Check sheet for the modelled part. Datum: model origin and axes. Units: mm. A direction names the side the tool comes from. Round coordinates to 2 decimals unless told otherwise and drop trailing zeros. Order: outer loops, then holes, each group sorted by start corner. A loop starts at its lowest first (then second) coordinate and runs counter-clockwise, first axis right, second up. Notation, with made-up numbers: M 55.5,-39.5 L 75.5,-39.5 A28 ccw 75.5,-19.5 Z; hole C 69,54 d7. An arc over 180 degrees is marked long. One line per item, written item: value. Start each with the question number.
(1) Access from +Z, -Z, +X, -X, +Y, -Y to the whole of each face (thin tool, end or side, straight path). Record for faces 1 (the face through (18, 24, 25)), 2 (the face through (9, 23, 12)).
(2) Depth check by flat-ended pin: pin 1 Ø3 at (x, y) = (19.5, 22.5) entering from +Z; pin 2 Ø7 at (x, z) = (6.5, 12) entering from -Y; pin 3 Ø8 at (y, z) = (12, 14) entering from -X; pin 4 Ø5 at (x, y) = (9, 19.5) entering from -Z. Enter the tip coordinate at first touch or a pass-through.
(3) Cross-section at B-B, the plane x = 12.5. Enter the section's corners in (y, z), and give its area (3 significant figures).
(4) Cross-section at A-A, the plane z = 12.5. Enter the section's corners in (x, y), and give its area (3 significant figures).
(5) Cross-section at D-D, the plane z = 2. Enter the section's corners in (x, y).
(6) Thickness scan on L1, parallel to Z at x = 12.5, y = 23.6; L2, parallel to Y at x = 13, z = 14.5. Record the ranges inside material, lowest first.
(7) Release check for a two-part mould opening along Z. For faces 3 (the face through (12.76, 24.014, 14.483)), 4 (the face through (23, 9, 12)), 5 (the face through (18, 24, 0)) record: released by +Z, released by -Z, zero draft, split by the parting line, or undercut.
from build123d import *

# Parameters (mm, degrees)
F1_DEPTH = 25
F2_R     = 2
F3_DEPTH = 25.001
F4_R     = 2
F5_DEPTH = 25.001


with BuildPart() as f1:
    # F0 (on Top) → F1 (new body)
    with BuildSketch(Plane.XY):
        Polygon((23, 23), (23, 0), (25, 0), (25, 25), (0, 25), (0, 23), align=None)
    extrude(amount=F1_DEPTH)

    # F2 (on face) → F3 (cut, through all)
    with BuildSketch(Plane(origin=(0, 25, 0), x_dir=(-1, 0, 0), z_dir=(0, 1, 0))):
        with Locations((-12.5, 12.5)):
            Circle(F2_R)
    extrude(amount=-F3_DEPTH, mode=Mode.SUBTRACT)

    # F4 (on face) → F5 (cut, through all)
    with BuildSketch(Plane.YZ.offset(25)):
        with Locations((12.5, 12.5)):
            Circle(F4_R)
    extrude(amount=-F5_DEPTH, mode=Mode.SUBTRACT)


solid = f1.part
Values found:
1. face 1: +Z, +X, -X, +Y, -Y
1. face 2: +Z, -Z, -X, -Y
2. pin 1: z = 25
2. pin 2: y = 23
2. pin 3: x = 23
2. pin 4: through
3. outline: M 23,0 L 25,0 L 25,10.5 L 23,10.5 Z; M 23,14.5 L 25,14.5 L 25,25 L 23,25 Z
3. area: 42.0 mm^2
4. outline: M 0,23 L 10.5,23 L 10.5,25 L 0,25 Z; M 14.5,23 L 23,23 L 23,14.5 L 25,14.5 L 25,25 L 14.5,25 Z; M 23,0 L 25,0 L 25,10.5 L 23,10.5 Z
4. area: 80.0 mm^2
5. outline: M 0,23 L 23,23 L 23,0 L 25,0 L 25,25 L 0,25 Z
6. L1: 0 to 10.5, 14.5 to 25
6. L2: 23 to 25
7. face 3: undercut
7. face 4: zero draft
7. face 5: released by -Z
